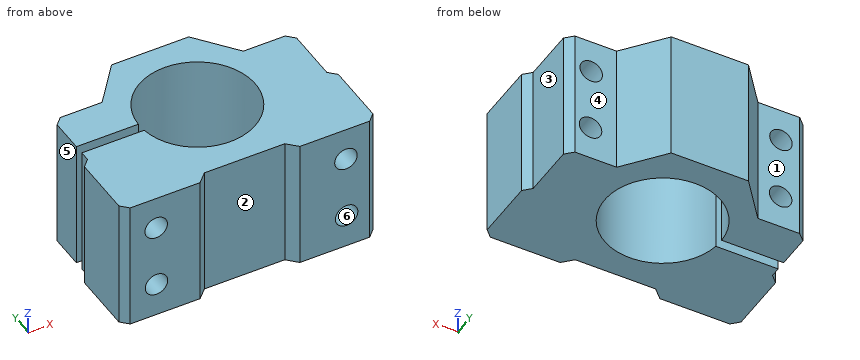
```python
from build123d import *

# Parameters (mm, degrees)
EXTRUDE_5_DEPTH     = 41
SKETCH_2_R          = 3.5
CUT_EXTRUDE_3_DEPTH = 50


with BuildPart() as part:
    # 草图1 → 凸台-拉伸5 (new body)
    with BuildSketch(Plane.XY):
        with BuildLine():
            ThreePointArc((21.653756169, 26.652324316), (57.479756353, 29.853440976), (21.511621785, 29.646721888))
            Line((21.511621785, 29.646721888), (2.250174694, 29.646721888))
            Line((2.250174694, 29.646721888), (2.250174694, 40.249825306))
            Line((2.250174694, 40.249825306), (4.500349388, 42.5))
            Line((4.500349388, 42.5), (17.500349388, 42.5))
            Line((17.500349388, 42.5), (27.5, 55))
            Line((27.5, 55), (51.5, 55))
            Line((51.5, 55), (61.4058809, 42.5))
            Line((61.4058809, 42.5), (74.4058809, 42.5))
            Line((74.4058809, 42.5), (76.70294045, 40.20294045))
            Line((76.70294045, 40.20294045), (76.70294045, 23.5941191))
            Line((76.70294045, 23.5941191), (79, 21.29705955))
            Line((79, 21.29705955), (79, 2.29705955))
            Line((79, 2.29705955), (76.70294045, 0))
            Line((76.70294045, 0), (55, 0))
            Line((55, 0), (52, 3))
            Line((52, 3), (27, 3))
            Line((27, 3), (24, 0))
            Line((24, 0), (2.250174694, 0))
            Line((2.250174694, 0), (0, 2.250174694))
            Line((0, 2.250174694), (0, 21.250174694))
            Line((0, 21.250174694), (2.250174694, 23.500349388))
            Line((2.250174694, 23.500349388), (2.250174694, 26.652324316))
            Line((2.250174694, 26.652324316), (21.653756169, 26.652324316))
        make_face()
    extrude(amount=EXTRUDE_5_DEPTH)

    # 草图2 → 切除-拉伸3 (cut)
    with BuildSketch(Plane(origin=(0, 0, 0), x_dir=(-1, 0, 0), z_dir=(0, -1, 0))):
        with Locations(Location((-10.435250124, -10.64238292, 0), (0, 0, 90))):
            Circle(SKETCH_2_R)
        with Locations(Location((-10.331990941, -30.64238292, 0), (0, 0, 90))):
            Circle(SKETCH_2_R)
        with Locations(Location((-69.331990941, -30.64238292, 0), (0, 0, 90))):
            Circle(SKETCH_2_R)
        with Locations(Location((-69.538509307, -10.64238292, 0), (0, 0, 90))):
            Circle(SKETCH_2_R)
    extrude(amount=-CUT_EXTRUDE_3_DEPTH, mode=Mode.SUBTRACT)


solid = part.part
```
The listing builds one solid part. Answer for the finished solid, in the listing's coordinates (mm). Face numbers are marked on the shaded views. A direction names the side the tool comes from. Round coordinates to 2 decimals unless told otherwise and drop trailing zeros. Loops run counter-clockwise (first coordinate to the right, second up) from the corner with the lowest first, then second, coordinate; pieces in that order, holes last. Notation, with made-up numbers: (-39, 23) -> (0, 23) arc R8 cw to (0, 31) -> close; hole circle Ø4 at (13, 66.25). An arc over 180 degrees is marked (long way). Use one line per item in the form item = value.
1. The part is cut by section D-D on y = 28.5. Determine the outline of the cut face in (x, z), and give its area (3 significant figures).
Answer key:
outline = (57.49, 0) -> (76.7, 0) -> (76.7, 41) -> (57.49, 41) -> close; hole circle Ø7 at (69.33, 30.64); hole circle Ø7 at (69.54, 10.64)
area = 711 mm²
2. For a pull along X with two mould halves and no side action, classify the marked faces 4, 5 and 6 as released by +X, released by -X, zero draft, split by the parting line, or undercut.
Answer key:
face_4 = zero draft
face_5 = released by -X
face_6 = undercut
3. The part is cut by section A-A on x = 39.5. Determine the outline of the cut face in (y, z).
Answer key:
outline = (3, 0) -> (11, 0) -> (11, 41) -> (3, 41) -> close; (47, 0) -> (55, 0) -> (55, 41) -> (47, 41) -> close
4. A tool of negligible diameter and unlimited length cuts with its end or side. For the marked faces 1, 2 and 3, from which of +Z, -Z, +X, -X, +Y, -Y can it reach the whole face along a straight path? Write none if from no direction.
Answer key:
face_1 = +Z, -Z, -X, +Y
face_2 = +Z, -Z, -Y
face_3 = +Z, -Z, +X, +Y
5. Flat-ended cylindrical pins translate along their axes: pin 1 Ø9 at (x, z) = (69.54, 10.64) entering from +Y; pin 2 Ø11.5 at (y, z) = (35, 14.5) entering from -X; pin 3 Ø7.5 at (x, z) = (38, 21.5) entering from -Y. Find the tip coordinate at first contact, or state that the pin passes through.
Answer key:
pin_1 = 42.5
pin_2 = 2.25
pin_3 = 3
6. The part is cut by section B-B on y = 38. Determine the outline of the cut face in (x, z), and give its area (3 significant figures).
Answer key:
outline = (2.25, 0) -> (23.91, 0) -> (23.91, 41) -> (2.25, 41) -> close; (55.09, 0) -> (76.7, 0) -> (76.7, 41) -> (55.09, 41) -> close; hole circle Ø7 at (10.33, 30.64); hole circle Ø7 at (10.44, 10.64); hole circle Ø7 at (69.33, 30.64); hole circle Ø7 at (69.54, 10.64)
area = 1,620 mm²
7. Find the intervals of material crossed by probe 1 along X at (y, z) = (22, 13); probe 2 along Z at (x, y) = (68, 37.5); probe 3 along X at (y, z) = (37, 8), in increasing order. Write a range as [from, to].
Answer key:
probe_1 = [0.75, 7.85], [13.02, 22.92], [56.08, 66.95], [72.13, 78.3]
probe_2 = [0, 7.5], [13.79, 27.41], [33.88, 41]
probe_3 = [2.25, 8.14], [12.73, 23.38], [55.62, 67.24], [71.83, 76.7]
8. The part is cut by section C-C on z = 21. Determine the outline of the cut face in (x, y), and give its area (3 significant figures).
Answer key:
outline = (0, 2.25) -> (2.25, 0) -> (24, 0) -> (27, 3) -> (52, 3) -> (55, 0) -> (76.7, 0) -> (79, 2.3) -> (79, 21.3) -> (76.7, 23.59) -> (76.7, 40.2) -> (74.41, 42.5) -> (61.41, 42.5) -> (51.5, 55) -> (27.5, 55) -> (17.5, 42.5) -> (4.5, 42.5) -> (2.25, 40.25) -> (2.25, 29.65) -> (21.51, 29.65) arc R18 cw (long way) to (21.65, 26.65) -> (2.25, 26.65) -> (2.25, 23.5) -> (0, 21.25) -> close
area = 2,520 mm²
